The model under review builds one solid part; all positions refer to its coordinate system, in mm. Round coordinates to 2 decimals unless told otherwise and drop trailing zeros. Write each loop counter-clockwise with the first axis right and the second up, starting at its lowest first coordinate (ties: lowest second). Pieces come first, ordered by that corner, then holes. Notation, with made-up numbers: (-6, 10.5) -> (-2, 10.5) arc R19 ccw to (-2, 40.5) -> close; hole circle Ø10 at (-12.5, 5). An arc over 180 degrees is marked (long way). Return JSON: item names as keys, results as strings. Group by question number.
1. Take a section at A-A, the plane x = 3. Write out the cut boundary in (y, z), then the cut area to 3 significant figures.
2. Clearance check with flat-ended pins moving along their axes: P1, Ø2.5, axis at x = 3, z = 0, coming from the +Y side; P2, Ø5, axis at x = -3, z = 0, coming from the +Y side. State where each tip first meets the part, or that it passes through.
3. Take a section at B-B, the plane z = 0. Write out the cut boundary in (x, y), then the cut area to 3 significant figures.
4. Mouldability with a two-part tool opening along X and no side actions: class faces 1 (the cylindrical face through (9.699, 0.887, 9.715)), 2 (the cylindrical face through (4.45, 0.32, 0.75)), 3 (the flat face through (0, 1.75, 0)) as pulls with the +X half, pulls with the -X half, needs draft (parallel to the pull), parting line crosses it, or undercut.
5. For line 1 along X through (y, z) = (0.2, 0); line 2 along X through (y, z) = (1.1, -1); line 3 along Z through (x, y) = (3.25, 0.5), list the stretches that pass through material, from the lowest coordinate up. Write a range as from..to.
from build123d import *

# Parameters (mm, degrees)
SKETCH1_W                                     = 20
SKETCH1_H                                     = 20
BOSS_EXTRUDE1_DEPTH                           = 1.75
CSK_FOR_4_FLAT_HEAD_MACHINE_SCREW1_AT_2_COUNT = 2
CSK_FOR_4_FLAT_HEAD_MACHINE_SCREW1_AT_2_PITCH = 6
FILLET2_R                                     = 1


with BuildPart() as part:
    # Sketch1 → Boss-Extrude1 (new body)
    with BuildSketch(Plane(origin=(0, 0, 0), x_dir=(1, 0, 0), z_dir=(0, 1, 0))):
        Rectangle(SKETCH1_W, SKETCH1_H)
    extrude(amount=BOSS_EXTRUDE1_DEPTH)

    # Sketch4 → CSK for #4 Flat Head Machine Screw1 (revolve, cut)
    with BuildSketch(Plane(origin=(3, 1.75, 0), x_dir=(0, 0, 1), z_dir=(1, 0, 0))):
        Polygon((0, 0), (0, 1.75), (1.63195, 1.75), (1.63195, 1.117640426), (2.6035, 0), align=None)
    csk_for_4_flat_head_machine_screw1 = revolve(axis=Axis((3, 8.1, 0), (0, -1, 0)), mode=Mode.SUBTRACT)

    # CSK for #4 Flat Head Machine Screw1 at 2: CSK for #4 Flat Head Machine Screw1 ×2
    with Locations(*[(-i * CSK_FOR_4_FLAT_HEAD_MACHINE_SCREW1_AT_2_PITCH, 0, 0) for i in range(1, CSK_FOR_4_FLAT_HEAD_MACHINE_SCREW1_AT_2_COUNT)]):
        add(csk_for_4_flat_head_machine_screw1, mode=Mode.SUBTRACT)

    # Fillet2
    fillet2_edges = [part.edges().sort_by_distance(p)[0] for p in [
        (10, 0.875, 10),
        (-10, 0.875, 10),
        (-10, 0.875, -10),
        (10, 0.875, -10),
    ]]
    fillet(fillet2_edges, radius=FILLET2_R)


solid = part.part
Output:
{
 "1": {"outline": "(0, -10) -> (1.75, -10) -> (1.75, -2.6) -> (0.63, -1.63) -> (0, -1.63) -> close; (0, 1.63) -> (0.63, 1.63) -> (1.75, 2.6) -> (1.75, 10) -> (0, 10) -> close", "area": "28.2 mm^2"},
 "2": {"P1": "passes through", "P2": "stops at y = 1.63"},
 "3": {"outline": "(-10, 0) -> (-4.63, 0) -> (-4.63, 0.63) -> (-5.6, 1.75) -> (-10, 1.75) -> close; (-1.37, 0) -> (1.37, 0) -> (1.37, 0.63) -> (0.4, 1.75) -> (-0.4, 1.75) -> (-1.37, 0.63) -> close; (4.63, 0) -> (10, 0) -> (10, 1.75) -> (5.6, 1.75) -> (4.63, 0.63) -> close", "area": "21.4 mm^2"},
 "4": {"face 1": "pulls with the +X half", "face 2": "undercut", "face 3": "needs draft"},
 "5": {"line 1": "x = -10..-4.63, -1.37..1.37, 4.63..10", "line 2": "x = -10..-4.78, -1.22..1.22, 4.78..10", "line 3": "z = -10..-1.61, 1.61..10"}
}
